Could you check a few things on this model? Use its own coordinates, in mm. Face numbers are marked on the shaded views. A direction names the side the tool comes from. Round coordinates to 2 decimals unless told otherwise and drop trailing zeros. Order: outer loops, then holes, each group sorted by start corner. A loop starts at its lowest first (then second) coordinate and runs counter-clockwise, first axis right, second up. Notation, with made-up numbers: (-30, -11.75) - (-1, -11.75) arc R17 cw to (-1, 1.25) - close; hole circle Ø10 at (7, 18). An arc over 180 degrees is marked (long way). Use one line per item in the form item = value.
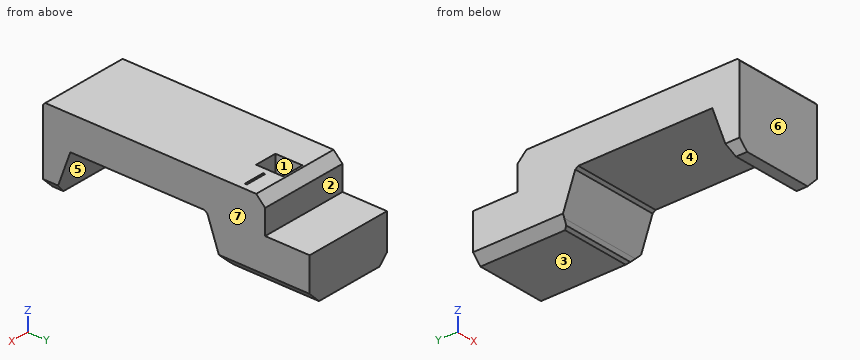
from build123d import *

# Parameters (mm, degrees)
BOSS_EXTRUDE1_DEPTH     = 400
SKETCH2_W               = 100
SKETCH2_H               = 121
SKETCH2_W_2             = 95.3
SKETCH2_H_2             = 9.4
CUT_EXTRUDE1_DEPTH      = 268
CUT_EXTRUDE2_DEPTH      = 1
CUT_EXTRUDE2_DEPTH_BACK = 1198.763658591


with BuildPart() as part:
    # Sketch1 → Boss-Extrude1 (new body)
    with BuildSketch(Plane(origin=(0, 0, 0), x_dir=(0, 0, -1), z_dir=(1, 0, 0))):
        Polygon((0, 0), (-340, 0), (-350, 10), (-350, 957.763658591), (-310, 997.763658591), (-200, 997.763658591), (-200, 1197.763658591), (-150, 1197.763658591), (0, 1197.763658591), (0, 997.763658591), (0, 967.763658591), (0, 817.763658591), (-9.396926208, 804.343457158), (-27.474774195, 797.763658591), (-190.603073792, 738.389813171), (-200, 724.969611738), (-200, 122.794046853), (0, 50), align=None)
    extrude(amount=BOSS_EXTRUDE1_DEPTH)

    # Sketch2 → Cut-Extrude1 (cut)
    with BuildSketch(Plane.XY.offset(350)):
        with Locations((200, 887.263658591)):
            Rectangle(SKETCH2_W, SKETCH2_H)
        with Locations((325, 887.263658591)):
            Rectangle(SKETCH2_W_2, SKETCH2_H_2)
    extrude(amount=-CUT_EXTRUDE1_DEPTH, mode=Mode.SUBTRACT)

    # Sketch3 → Cut-Extrude2 (cut, two sides)
    with BuildSketch(Plane(origin=(0, 0, 0), x_dir=(-1, 0, 0), z_dir=(0, -1, 0))) as cut_extrude2_sk:
        Polygon((32.971910004, -72.804395349), (-67.728153305, 29.569560354), (-322.648629759, 29.569560354), (-423.348693067, -72.804395349), (-423.348693067, 100.069531779), (32.971910004, 100.069531779), align=None)
    extrude(amount=CUT_EXTRUDE2_DEPTH, mode=Mode.SUBTRACT)
    extrude(cut_extrude2_sk.sketch, amount=-CUT_EXTRUDE2_DEPTH_BACK, mode=Mode.SUBTRACT)


solid = part.part
Item 1: Imagine slicing it at C-C on x = 237.5. Please give me the cut outline in (y, z).
Found:
outline = (0, 0) - (50, 0) - (122.79, 200) - (724.97, 200) - (738.39, 190.6) - (804.34, 9.4) - (817.76, 0) - (1197.76, 0) - (1197.76, 200) - (997.76, 200) - (997.76, 310) - (957.76, 350) - (947.76, 350) - (947.76, 82) - (826.76, 82) - (826.76, 350) - (10, 350) - (0, 340) - close
Item 2: Imagine slicing it at B-B on z = 286.5. Please give me the cut outline in (x, y).
Found:
outline = (0, 0) - (400, 0) - (400, 997.76) - (0, 997.76) - close; hole (150, 826.76) - (250, 826.76) - (250, 947.76) - (150, 947.76) - close; hole (277.35, 882.56) - (372.65, 882.56) - (372.65, 891.96) - (277.35, 891.96) - close
Item 3: Imagine slicing it at D-D on y = 449.5. Please give me the cut outline in (x, z), plus the area to 3 significant figures.
Found:
outline = (0, 200) - (400, 200) - (400, 350) - (0, 350) - close
area = 60,000 mm2
Item 4: Imagine slicing it at A-A on z = 167.5. Please give me the cut outline in (x, y), plus the area to 3 significant figures.
Found:
outline = (0, 0) - (400, 0) - (400, 110.97) - (0, 110.97) - close; (0, 746.8) - (400, 746.8) - (400, 1197.76) - (0, 1197.76) - close; hole (150, 826.76) - (250, 826.76) - (250, 947.76) - (150, 947.76) - close; hole (277.35, 882.56) - (372.65, 882.56) - (372.65, 891.96) - (277.35, 891.96) - close
area = 212,000 mm2
Item 5: I need wall thicknesses on L1, parallel to Y at x = 156, z = 146; L2, parallel to Y at x = 228, z = 184.5; L3, parallel to Y at x = 229.5, z = 233.5. Which ranges of each line are inside material? Lowest first, please.
Found:
L1 = 0 to 103.14, 754.62 to 826.76, 947.76 to 1197.76
L2 = 0 to 117.15, 740.61 to 826.76, 947.76 to 1197.76
L3 = 0 to 826.76, 947.76 to 997.76
Item 6: Will these pins go through, and if not, where does the flat tip stop? P1, Ø1.5, axis at x = 110, y = 644.5, coming from the -Z side; P2, Ø7.5, axis at x = 321.5, y = 888, coming from the +Z side.
Found:
P1 = 200
P2 = 82
Item 7: If we mould it in two halves opening along Y, with no side actions, what happens to the marked faces 5, 6 and 7? For each: released by +Y, released by -Y, zero draft, split by the parting line, or undercut.
Found:
face_5 = undercut
face_6 = released by -Y
face_7 = zero draft
Item 8: For the marked faces 1, 2, 3 and 4, which set-ups out of +Z, -Z, +X, -X, +Y, -Y let a thin tool reach every point of the face, with its end or its side?
Found:
face_1 = +Z
face_2 = +Z, +X, -X, +Y
face_3 = -Z, +X, -X, +Y, -Y
face_4 = -Z, +X, -X
